Here's how the part is built. I have some questions about the finished solid (model axes, mm). Round coordinates to 2 decimals unless told otherwise and drop trailing zeros. Loops run counter-clockwise (first coordinate to the right, second up) from the corner with the lowest first, then second, coordinate; pieces in that order, holes last. Notation, with made-up numbers: M 0,29 L 10,29 A24 ccw 10,68 Z; hole C 15.25,61 d11. An arc over 180 degrees is marked long. Answer as CSV lines item,"result".
```python
from build123d import *

# Parameters (mm, degrees)
WANDUNG1_T                           = -2
SCHNITT_LINEAR_AUSTRAGEN1_DEPTH      = 56.901699437
SCHNITT_LINEAR_AUSTRAGEN1_DEPTH_BACK = 56.901699437
SKIZZE3_R                            = 10


with BuildPart() as part:
    # Aufsatz-Linear austragen1 cone 1 section (through the dimple's axis) → Aufsatz-Linear austragen1 (revolve)
    with BuildSketch(Plane(origin=(0, 0, 0), x_dir=(0, -1, 0), z_dir=(1, 0, 0))):
        Polygon((0, 0), (25, 0), (0, 43.301270189), align=None)
    revolve(axis=Axis((0, 0, 0), (0, 0, -1)))

    # Wandung1
    wandung1_openings = [part.faces().sort_by_distance(p)[0] for p in [
        (0, 0, 0),
    ]]
    offset(amount=WANDUNG1_T, openings=wandung1_openings, kind=Kind.INTERSECTION)

    # Skizze3 → Schnitt-Linear austragen1 (cut, two sides: drawn at the far end of the back side and taken through both)
    with BuildSketch(Plane.XY.offset(-SCHNITT_LINEAR_AUSTRAGEN1_DEPTH_BACK)):
        Circle(SKIZZE3_R)
    extrude(amount=SCHNITT_LINEAR_AUSTRAGEN1_DEPTH + SCHNITT_LINEAR_AUSTRAGEN1_DEPTH_BACK, mode=Mode.SUBTRACT)


solid = part.part
```
1. We'd pull the mould along Y, two halves only. Please class faces 1 (the flat face through (20.3, 11, 0)), 2 (the conical face through (7.32, 9.54, -18.47)), 3 (the conical face through (-3.723, -11.823, -21.833)): pulls with the +Y half, pulls with the -Y half, needs draft (parallel to the pull), parting line crosses it, or undercut.
Evaluation:
face 1,"needs draft"
face 2,"undercut"
face 3,"parting line crosses it"
2. For P1, Ø1, axis at x = -6, y = -11.5, coming from the +Z side; P2, Ø10, axis at y = 5, z = -21, coming from the +X side; P3, Ø2, axis at x = 2, z = -14, coming from the +Y side; P4, Ø1, axis at x = -8.5, y = -1.5, coming from the +Z side, each with a flat end and sliding along its axis, tell me the tip position at first contact or that it passes through.
Evaluation:
P1,"stops at z = -15.97"
P2,"stops at x = 15.24"
P3,"stops at y = 17.39"
P4,"passes through"
3. I want a section at C-C, the plane z = -16.5. Please give me the cut outline in (x, y), and give its area (3 significant figures).
Evaluation:
outline,"C 0,0 d30.95; hole C 0,0 d26.33"
area,"208 mm²"
4. I want a section at A-A, the plane y = 0. Please give me the cut outline in (x, z).
Evaluation:
outline,"M -25,0 L -10,-25.98 L -10,-21.98 L -22.69,0 Z; M 10,-25.98 L 25,0 L 22.69,0 L 10,-21.98 Z"
5. If I drill on line 1 (Y direction, x = -4.5, z = -22); line 2 (X direction, y = 0, z = -24.45); line 3 (Y direction, x = 0, z = -24.7), over which ranges is the centre line in solid material (lowest first)? Write a range as [from, to].
Evaluation:
line 1,"y = [-11.45, -8.93], [8.93, 11.45]"
line 2,"x = [-10.88, -10], [10, 10.88]"
line 3,"y = [-10.74, -10], [10, 10.74]"
